from build123d import *

# Parameters (mm, degrees)
BOSS_EXTRUDE1_DEPTH = 26
SKETCH2_R           = 1.7
CUT_EXTRUDE1_DEPTH  = 31
CUT_EXTRUDE2_DEPTH  = 1


with BuildPart() as part:
    # Sketch1 → Boss-Extrude1 (new body)
    with BuildSketch(Plane(origin=(0, 0, 0), x_dir=(1, 0, 0), z_dir=(0, 1, 0))):
        with BuildLine():
            Line((-46.998275301, 32.528571429), (-46.998275301, -39.471428571))
            Line((-46.998275301, -39.471428571), (-16.998275301, -39.471428571))
            Line((-16.998275301, -39.471428571), (-16.998275301, -27.471428571))
            ThreePointArc((-16.998275301, -27.471428571), (-40.998275301, -3.471428571), (-16.998275301, 20.528571429))
            Line((-16.998275301, 20.528571429), (-16.998275301, 32.528571429))
            Line((-16.998275301, 32.528571429), (-46.998275301, 32.528571429))
        make_face()
    extrude(amount=BOSS_EXTRUDE1_DEPTH)

    # Sketch2 → Cut-Extrude1 (cut, through all)
    with BuildSketch(Plane(origin=(-16.998275301, 0, 0), x_dir=(0, 0, -1), z_dir=(1, 0, 0))):
        with Locations((-34.471428571, 13)):
            Circle(SKETCH2_R)
        with Locations((27.528571429, 13)):
            Circle(SKETCH2_R)
    extrude(amount=-CUT_EXTRUDE1_DEPTH, mode=Mode.SUBTRACT)

    # Sketch3 → Cut-Extrude2 (cut)
    with BuildSketch(Plane(origin=(-16.998275301, 0, 0), x_dir=(0, 0, -1), z_dir=(1, 0, 0))):
        Polygon((-34.164231178, 21.664809495), (-32.617436306, 21.664809495), (-32.617436306, 21.33916847), (-33.87929528, 21.33916847), (-33.87929528, 20.362245393), (-32.617436306, 20.362245393), (-32.617436306, 20.036604367), (-33.87929528, 20.036604367), (-33.87929528, 18.489809495), (-34.164231178, 18.489809495), align=None)
        Polygon((-30.599352372, 21.746219752), (-30.541474768, 21.746219752), (-30.541474768, 19.548142829), (-30.175128614, 19.548142829), (-30.175128614, 19.222501803), (-30.541474768, 19.222501803), (-30.541474768, 18.489809495), (-30.826410665, 18.489809495), (-30.826410665, 19.222501803), (-32.332500409, 19.222501803), align=None)
        Polygon((-30.826410665, 19.548142829), (-30.826410665, 20.925757011), (-31.772168878, 19.548142829), align=None, mode=Mode.SUBTRACT)
    extrude(amount=-CUT_EXTRUDE2_DEPTH, mode=Mode.SUBTRACT)


solid = part.part
Work out the finished part from the listing and answer in its coordinate system (mm). Round coordinates to 2 decimals unless told otherwise and drop trailing zeros. Order: outer loops, then holes, each group sorted by start corner. A loop starts at its lowest first (then second) coordinate and runs counter-clockwise, first axis right, second up. Notation, with made-up numbers: M 83.25,-38.5 L 108.25,-38.5 A23 ccw 108.25,-23.5 Z; hole C -13,17.25 d8. An arc over 180 degrees is marked long. One line per item, written item: value.
Q1. Find section B-B on y = 13. Write down the section's boundary in (x, z).
Derived:
outline: M -47,-32.53 L -17,-32.53 L -17,-29.23 L -47,-29.23 Z; M -47,-25.83 L -17,-25.83 L -17,-20.53 A24 cw -17,27.47 L -17,32.77 L -47,32.77 Z; M -47,36.17 L -17,36.17 L -17,39.47 L -47,39.47 Z
Q2. Find section D-D on y = 5. Write down the section's boundary in (x, z), then the cut area to 3 significant figures.
Derived:
outline: M -47,-32.53 L -17,-32.53 L -17,-20.53 A24 cw -17,27.47 L -17,39.47 L -47,39.47 Z
area: 1,260 mm²
Q3. Flat-ended cylindrical pins translate along their axes: pin 1 (0.5 mm diameter, centred on x = -17.5, z = 33, fed in from -Y); pin 2 (8 mm diameter, centred on y = 20, z = -6.5, fed in from +X). Find the tip coordinate at first contact, or state that the pin passes through.
Derived:
pin 1: y = 0
pin 2: x = -36.51
Q4. Find section A-A on x = -20. Write down the section's boundary in (y, z).
Derived:
outline: M 0,-32.53 L 26,-32.53 L 26,-20.34 L 0,-20.34 Z; M 0,27.28 L 26,27.28 L 26,39.47 L 0,39.47 Z; hole C 13,-27.53 d3.4; hole C 13,34.47 d3.4
Q5. Determine the mould class of faces 1 (the face through (-32, 13, -32.529)), 2 (the face through (-42, 26, 3)), 3 (the face through (-31.79, 13.51, -29.15)) for opening direction Z: released by +Z, released by -Z, zero draft, split by the parting line, or undercut.
Derived:
face 1: released by -Z
face 2: zero draft
face 3: undercut
Q6. Find section C-C on x = -32.5. Write down the section's boundary in (y, z).
Derived:
outline: M 0,-32.53 L 26,-32.53 L 26,-14.85 L 0,-14.85 Z; M 0,21.79 L 26,21.79 L 26,39.47 L 0,39.47 Z; hole C 13,-27.53 d3.4; hole C 13,34.47 d3.4
Q7. Straight lines are drawn through the part: line 1 (Z direction, x = -44.25, y = 12.25); line 2 (Z direction, x = -36.25, y = 12.25); line 3 (Y direction, x = -33.5, z = 33.5). For each, find the intervals that lie inside material, in ascending order.
Derived:
line 1: -32.53 to -29.05, -26 to 32.95, 36 to 39.47
line 2: -32.53 to -29.05, -26 to -10.86, 17.8 to 32.95, 36 to 39.47
line 3: 0 to 11.6, 14.4 to 26
